Autodesk Inventor part; units mm, degrees
ref_plane "Work Plane3" through (-6.9376, -3.175, 8.1734) normal (0, -1, 0) x (1, 0, 0)
ref_plane "YZ Plane" through (0, 0, 0) normal (1, 0, 0) x (0, 1, 0)
ref_plane "XZ Plane" through (0, 0, 0) normal (0, 1, 0) x (-1, 0, 0)
sketch "Sketch1" plane through (0, 0, 0) normal (0, 0, 1) x (1, 0, 0)
  circle A0 centre (0, 0) radius 7
  line L0 (-2.5, -9) -> (-2.5, -6.5383)
  line L1 (-2.5, -9) -> (2.5, -9)
  line L2 (-2.5, -9) -> (-2.5, -6.5383)
  line L3 (2.5, -6.5383) -> (2.5, -9)
  circle A1 centre (0, 0) radius 12.5
  dimension "d0" = 25
extrude "Extrusion1" add sketch "Sketch1" against normal blind 20
sketch "Sketch2" plane through (0, 0, 0) normal (0, 0, 1) x (1, 0, 0)
  circle A0 centre (0, 0) radius 12.5
extrude "Extrusion2" add sketch "Sketch2" along normal blind 8
sketch "Sketch3" plane through (0, 0, 8) normal (0, 0, 1) x (1, 0, 0)
  circle A0 centre (0, 0) radius 12.5
  line L0 (2.433, -3.175) -> (-2.433, -3.175)
  arc A1 (2.433, -3.175) -> (-2.433, -3.175) centre (0, 0) ccw
extrude "Extrusion3" add sketch "Sketch3" along normal blind 12
ref_plane "Work Plane2" through (0, -12.5, 0) normal (0, -1, 0) x (1, 0, 0)
ref_plane "Work Plane1" through (2.433, -3.175, 10) normal (0, -1, 0) x (-1, 0, 0)
sketch "Sketch4" plane through (0, -12.5, 0) normal (0, -1, 0) x (1, 0, 0)
  line L0 (12.5, 20) -> (-12.5, 20)
  circle A0 centre (0, 12) radius 3
  point P0 (0, 0)
  dimension "d7" = 6
  dimension "d8" = 8
ref_plane "Work Plane3" through (-6.9376, -3.175, 8.1734) normal (0, -1, 0) x (1, 0, 0)
extrude "Extrusion4" cut sketch "Sketch4" against normal up to surface (9.325 mm away)
thread "Thread1"
properties part number "nmrv-50 to mega torque mototr coupler"
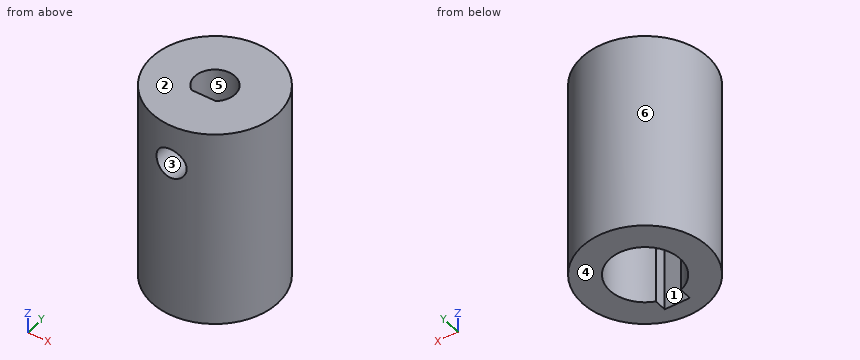
Could you check a few things on this model? Use its own coordinates, in mm. Face numbers are marked on the shaded views. A direction names the side the tool comes from. Coordinates: 2 decimals unless noted, no trailing zeros. Order: outer loops, then holes, each group sorted by start corner. A loop starts at its lowest first (then second) coordinate and runs counter-clockwise, first axis right, second up. Notation, with made-up numbers: (-2, 32) - (46, 32) arc R21 ccw to (46, 36) - close; hole circle Ø9 at (-39.75, 73.25). An arc over 180 degrees is marked (long way). Answer in a Markdown table with one row per item. Add a question column.
(1) If we section it at A-A, the plane x = 0: Please give me the cut outline in (y, z) (3 decimals).
(2) If we section it at C-C, the plane y = -8.25: Please give me the cut outline in (x, z), then the cut area to 3 significant figures.
(3) If we section it at B-B, the plane y = 0: Please give me the cut outline in (x, z), then the cut area to 3 significant figures.
(4) Will these pins go through, and if not, where does the flat tip stop? pin 1 (2.5 mm diameter, centred on y = -7.5, z = -12.5, fed in from +X); pin 2 (10 mm diameter, centred on y = -2, z = -2.5, fed in from -X); pin 3 (2 mm diameter, centred on x = -3.5, z = 6.5, fed in from -Y); pin 4 (2.5 mm diameter, centred on y = -7, z = -14.5, fed in from -X).
(5) On a 3-axis mill with a long thin cutter (end or side, diameter ignored), from which of +Z, -Z, +X, -X, +Y, -Y can I reach the whole of each face in a straight line? I mean the marked faces 1, 2 and 3. Say none if no direction works.
(6) I need wall thicknesses on L1, parallel to Y at x = 0, z = -12.5; L2, parallel to Z at x = -4.5, y = -1.5; L3, parallel to X at y = 2.25, z = -15. Which ranges of each line are inside material? Lowest first, please.
(7) If we section it at D-D, the plane z = 17: Please give me the cut outline in (x, y) (3 decimals).
(8) If we mould it in two halves opening along X, with no side actions, what happens to the marked faces 4, 5 and 6? For each: released by +X, released by -X, zero draft, split by the parting line, or undercut.
Results are:
| question | item | result |
|---|---|---|
| 1 | outline | (-12.5, -20) - (-9, -20) - (-9, 0) - (7, 0) - (7, -20) - (12.5, -20) - (12.5, 20) - (4, 20) - (4, 8) - (-3.175, 8) - (-3.175, 9) - (-12.5, 9) - close; (-12.5, 15) - (-3.175, 15) - (-3.175, 20) - (-12.5, 20) - close |
| 2 | outline | (-9.39, -20) - (-2.5, -20) - (-2.5, 0) - (2.5, 0) - (2.5, -20) - (9.39, -20) - (9.39, 20) - (-9.39, 20) - close; hole circle Ø6 at (0, 12) |
| 2 | area | 623 mm2 |
| 3 | outline | (-12.5, -20) - (-7, -20) - (-7, 0) - (7, 0) - (7, -20) - (12.5, -20) - (12.5, 20) - (4, 20) - (4, 8) - (-4, 8) - (-4, 20) - (-12.5, 20) - close |
| 3 | area | 624 mm2 |
| 4 | pin 1 | stops at x = 10.83 |
| 4 | pin 2 | stops at x = -12.5 |
| 4 | pin 3 | stops at y = -12.25 |
| 4 | pin 4 | stops at x = -11.1 |
| 5 | face 1 | -Z |
| 5 | face 2 | +Z, +X, -X, +Y, -Y |
| 5 | face 3 | -Y |
| 6 | L1 | y = -12.5 to -9, 7 to 12.5 |
| 6 | L2 | z = 0 to 20 |
| 6 | L3 | x = -12.3 to -6.63, 6.63 to 12.3 |
| 7 | outline | circle Ø25 at (0, 0); hole (-2.433, -3.175) - (2.433, -3.175) arc R4 ccw (long way) to start |
| 8 | face 4 | zero draft |
| 8 | face 5 | undercut |
| 8 | face 6 | split by the parting line |
